Autodesk Inventor part; units mm, degrees
ref_plane "YZ Plane" through (0, 0, 0) normal (1, 0, 0) x (0, 1, 0)
ref_plane "XZ Plane" through (0, 0, 0) normal (0, 1, 0) x (-1, 0, 0)
ref_plane "XY Plane" through (0, 0, 0) normal (0, 0, 1) x (1, 0, 0)
sketch "Esquisse1" plane through (0, 0, 0) normal (1, 0, 0) x (0, 1, 0)
  line L0 (0, 0) -> (60, 0)
  line L1 (60, 0) -> (60, -50)
  line L2 (60, -50) -> (0, -50)
  line L3 (0, -50) -> (0, 0)
  dimension "d0" = 60
  dimension "d1" = 50
extrude "Extrusion1" add sketch "Esquisse1" along normal blind 110
shell "Coque1" thickness 1 removed faces 1 at (36.6667, 0, -33.3333)
sketch "Esquisse2" plane through (0, 0, -50) normal (0, -1, 0) x (1, 0, 0)
  line L0 (0, 50) -> (110, 50)
  line L1 (110, 0) -> (110, 50)
  line L2 (110, 50) -> (110, 0)
  line L3 (110, 25) -> (110, 19)
  line L4 (110, 25) -> (110, 31)
  line L5 (0, 50) -> (0, 0)
  line L6 (84, 19) -> (61.25, 19)
  line L7 (84, 31) -> (61.25, 31)
  line L8 (110, 50) -> (0, 50)
  line L9 (0, 50) -> (0, 0)
  line L10 (0, 0) -> (110, 0)
  line L11 (0, 0) -> (110, 0)
  line L12 (109, 49) -> (109, 1)
  line L13 (110, 31) -> (110, 19)
  line L14 (110, 50) -> (110, 0)
  line L15 (61.25, 31) -> (57.25, 31)
  line L16 (57.25, 31) -> (57.25, 19)
  line L17 (82.25, 19) -> (86.25, 19)
  line L18 (109, 31) -> (105, 31)
  line L19 (80, 31) -> (80, 19)
  line L20 (1, 49) -> (109, 49)
  line L21 (57.25, 19) -> (61.25, 19)
  line L22 (110, 50) -> (80, 50)
  line L23 (0, 50) -> (110, 50)
  line L24 (80, 31) -> (80, 50)
  dimension "d5" = 6
  dimension "d6" = 6
  dimension "d7" = 48.75
  dimension "d50" = 4
  dimension "d67" = 30
extrude "Extrusion2" add sketch "Esquisse2" along normal blind 1
sketch "Esquisse3" plane through (0, 0, 0) normal (-1, 0, 0) x (0, 0, 1)
  line L0 (0, 0) -> (-19, 0)
  line L1 (-19, 0) -> (-19, 10)
  line L2 (-19, 10) -> (-31, 10)
  line L3 (-31, 10) -> (-31, 33.75)
  line L4 (-31, 33.75) -> (-19, 33.75)
  line L5 (-19, 33.75) -> (-19, 10)
  dimension "d10" = 10
  dimension "d11" = 12
  dimension "d12" = 23.75
extrude "Extrusion3" cut sketch "Esquisse3" against normal blind 1
sketch "Esquisse4" plane through (110, 60, -50) normal (0, 0, -1) x (-1, 0, 0)
  line L0 (110, -61) -> (110, 0)
  line L1 (110, -61) -> (100, -61)
  line L2 (0, -61) -> (110, -61)
  line L3 (110, 0) -> (0, 0)
  circle A0 centre (80, -50.5) radius 4
  line L4 (110, 0) -> (0, 0)
  circle A1 centre (80, -10.5) radius 4
  line L5 (110, 0) -> (80, 0)
  line L6 (80, -10.5) -> (80, -50.5)
  line L7 (80, -50.5) -> (80, -61)
  point P0 (110, -60)
  dimension "d15" = 10
  dimension "d28" = 8
  dimension "d48" = 8
  dimension "d65" = 30
  dimension "d69" = 40
  dimension "d70" = 10.5
extrude "Extrusion4" add sketch "Esquisse4" along normal blind 3
sketch "Esquisse8" plane through (0, 60, 0) normal (0, 0, 1) x (1, 0, 0)
  circle A0 centre (30, -10.5) radius 4
  line L0 (110, -61) -> (0, -61)
  circle A1 centre (30, -50.5) radius 4
  circle A2 centre (30, -50.5) radius 4
  line L1 (30, -21.5) -> (30, -14.5)
  line L2 (30, -44.5) -> (30, -46.5)
  line L3 (0, -61) -> (0, 0)
  line L4 (0, 0) -> (30, 0)
  line L5 (0, 0) -> (110, 0)
  line L6 (30, -50.5) -> (30, -10.5)
  line L7 (1, -1) -> (109, -1)
  line L8 (30, -10.5) -> (30, 0)
  line L9 (30, -50.5) -> (30, -61)
  point P0 (0, -60)
  point P1 (30, -6.5)
  dimension "d74" = 8
  dimension "d40" = 8
  dimension "d66" = 30
  dimension "d73" = 40
extrude "Extrusion8" add sketch "Esquisse8" along normal blind 3 contours L6 L8 A0 | A0 L8 L6 | L6 L9 A1 | A1 L9 L6
sketch "Esquisse6" plane through (0, 60, 0) normal (0, 1, 0) x (1, 0, 0)
  line L0 (1, 49) -> (109, 49)
  line L1 (1, 1) -> (1, 49)
  line L2 (1, 49) -> (109, 49)
  line L3 (109, 49) -> (109, 1)
  line L4 (109, 1) -> (1, 1)
  line L5 (110, 0) -> (0, 0)
extrude "Extrusion6" cut sketch "Esquisse6" against normal blind 10
sketch "Esquisse12" plane through (0, 60, 0) normal (0, 0, 1) x (1, 0, 0)
  line L0 (110, 0) -> (110, -61)
  line L1 (110, 0) -> (97, 0)
  line L2 (1, 0) -> (109, 0)
  line L3 (97, 0) -> (97, -17.5)
  circle A0 centre (97, -17.5) radius 7.8
  line L4 (97, -17.5) -> (97, -43.5)
  circle A1 centre (97, -43.5) radius 7.8
  point P0 (0, -60)
  dimension "d51" = 13
  dimension "d52" = 17.5
  dimension "d53" = 15.6
  dimension "d54" = 26
  dimension "d55" = 15.6
extrude "Extrusion9" cut sketch "Esquisse12" against normal through all
sketch "Esquisse13" plane through (0, -1, -50) normal (0, -1, 0) x (1, 0, 0)
  line L0 (0, 0) -> (110, 0)
  line L1 (110, 0) -> (97, 0)
  line L2 (97, 0) -> (97, 12)
  line L3 (97, 12) -> (97, 38)
  line L4 (97, 38) -> (97, 50)
  circle A0 centre (97, 38) radius 7.85
  circle A1 centre (97, 12) radius 7.85
  point P0 (0, 50)
  dimension "d58" = 13
  dimension "d59" = 12
  dimension "d60" = 26
  dimension "d61" = 15.7
  dimension "d62" = 15.7
extrude "Extrusion10" cut sketch "Esquisse13" against normal blind 10
properties part number "Torse"
Here's how the part is built. I have some questions about the finished solid (model axes, mm). A direction names the side the tool comes from. Give positions to 0.01 mm unless a question says otherwise; leave off trailing zeros. Loops run counter-clockwise (first coordinate to the right, second up) from the corner with the lowest first, then second, coordinate; pieces in that order, holes last. Notation, with made-up numbers: (-24.75, 4.25) -> (-19.75, 4.25) arc R10 cw to (-19.75, 22.25) -> close; hole circle Ø11 at (19.5, 65). An arc over 180 degrees is marked (long way). Use one line per item in the form item = value. Start each with the question number.
1) Please list where these lines run through material, in increasing order: line 1 along Y through (x, z) = (97, -49.7); line 2 along Z through (x, y) = (35, 7.5); line 3 along X through (y, z) = (39, -37.5).
2) Imagine slicing it at C-C (z = -12). Please give me the cut outline in (x, y), then the cut area to 3 significant figures.
3) For P1, Ø25, axis at x = 97, y = 16.5, coming from the +Z side; P2, Ø0.8, axis at x = 69, y = -0.5, coming from the -Z side; P3, Ø12, axis at x = 92.5, z = -9, coming from the +Y side; P4, Ø12.5, axis at x = 97, z = -38, coming from the -Y side, each with a flat end and sliding along its axis, tell me the tip position at first contact or that it passes through.
4) Imagine slicing it at D-D (x = 77). Please give me the cut outline in (y, z), then the cut area to 3 significant figures.
5) Which directions (+Z, -Z, +X, -X, +Y, -Y) give clear straight access to the entire face, cutting with the end or side of a thin tool? Please do faces 4 (the face through (110, 29, -25)), 5 (the face through (42, 0, -25)).
6) Thinking about a two-plate mould opening in X: for faces 1 (the face through (56, 30, -1)), 2 (the face through (26.8, 11.9, 1.5)), 3 (the face through (54, 29, 0)), which applies, +X half, -X half, draft (parallel to the pull), parting line (faces both ways), or undercut?
7) Imagine slicing it at A-A (y = 16.5). Please give me the cut outline in (x, z).
8) Imagine slicing it at B-B (x = 14). Please give me the cut outline in (y, z), then the cut area to 3 significant figures.
Check values:
q1.line_1 = -1 to 8.7, 24.3 to 34.7, 50.3 to 60
q1.line_2 = -50 to -49, -1 to 0
q1.line_3 = 0 to 1, 109 to 110
q2.outline = (0, -1) -> (89.15, -1) -> (89.15, 0) -> (1, 0) -> (1, 60) -> (0, 60) -> close; (104.85, -1) -> (110, -1) -> (110, 60) -> (109, 60) -> (109, 0) -> (104.85, 0) -> close
q2.area = 214 mm^2
q3.P1 = 0
q3.P2 = -50
q3.P3 = 0
q3.P4 = through
q4.outline = (-1, -50) -> (60, -50) -> (60, -49) -> (0, -49) -> (0, -31) -> (-1, -31) -> close; (-1, -19) -> (0, -19) -> (0, -1) -> (60, -1) -> (60, 0) -> (-1, 0) -> close
q4.area = 158 mm^2
q5.face_4 = +Z, -Z, +X, +Y, -Y
q5.face_5 = +Y
q6.face_1 = undercut
q6.face_2 = parting line
q6.face_3 = draft
q7.outline = (0, -50) -> (89.2, -50) -> (89.2, -49) -> (1, -49) -> (1, -31) -> (0, -31) -> close; (0, -19) -> (1, -19) -> (1, -1) -> (89.2, -1) -> (89.2, 0) -> (0, 0) -> close; (104.8, -50) -> (110, -50) -> (110, 0) -> (104.8, 0) -> (104.8, -1) -> (109, -1) -> (109, -49) -> (104.8, -49) -> close
q8.outline = (-1, -50) -> (60, -50) -> (60, -49) -> (0, -49) -> (0, -1) -> (60, -1) -> (60, 0) -> (-1, 0) -> close
q8.area = 170 mm^2
